Source: CAD feature listing. Evaluate the final solid. Frame: model axes, mm. A direction names the side the tool comes from. Give positions to 0.01 mm unless a question says otherwise; leave off trailing zeros. Loops run counter-clockwise (first coordinate to the right, second up) from the corner with the lowest first, then second, coordinate; pieces in that order, holes last.
from build123d import *

# Parameters (mm, degrees)
SKETCH1_R               = 1.55
BOSS_EXTRUDE1_DEPTH     = 7
SKETCH2_R               = 2.75
CUT_EXTRUDE1_DEPTH      = 5
SKETCH3_R               = 1.75
CUT_EXTRUDE2_DEPTH      = 5
CUT_EXTRUDE4_DEPTH      = 7
CUT_EXTRUDE4_DEPTH_BACK = 7
FILLET1_R               = 10


with BuildPart() as part:
    # Sketch1 → Boss-Extrude1 (new body)
    with BuildSketch(Plane.XY):
        with BuildLine():
            ThreePointArc((0, 6), (-6, 0), (0, -6))
            Line((0, -6), (44.5, -4))
            ThreePointArc((44.5, -4), (48.5, 0), (44.5, 4))
            Line((44.5, 4), (0, 6))
        make_face()
        with Locations((44.5, 0)):
            Circle(SKETCH1_R, mode=Mode.SUBTRACT)
    extrude(amount=BOSS_EXTRUDE1_DEPTH)

    # Sketch2 → Cut-Extrude1 (cut)
    with BuildSketch(Plane.XY.offset(7)):
        Circle(SKETCH2_R)
    extrude(amount=-CUT_EXTRUDE1_DEPTH, mode=Mode.SUBTRACT)

    # Sketch3 → Cut-Extrude2 (cut)
    with BuildSketch(Plane(origin=(0, 0, 0), x_dir=(-1, 0, 0), z_dir=(0, 0, -1))):
        Circle(SKETCH3_R)
    extrude(amount=-CUT_EXTRUDE2_DEPTH, mode=Mode.SUBTRACT)

    # Sketch5 → Cut-Extrude4 (cut, two sides)
    with BuildSketch(Plane(origin=(0, 0, 0), x_dir=(1, 0, 0), z_dir=(0, 1, 0))) as cut_extrude4_sk:
        with BuildLine():
            Line((48.5, 0), (48.5, -2.5))
            Line((48.5, -2.5), (28.5, -2.5))
            add(Edge.make_bspline(
                [(9, 0), (9.734542775, -1.732075598), (8.772191405, -2.578671179), (28.5, -2.5)],
                knots=[0, 0, 0, 0, 1, 1, 1, 1], degree=3))
            Line((9, 0), (48.5, 0))
        make_face()
    extrude(amount=CUT_EXTRUDE4_DEPTH, mode=Mode.SUBTRACT)
    extrude(cut_extrude4_sk.sketch, amount=-CUT_EXTRUDE4_DEPTH_BACK, mode=Mode.SUBTRACT)

    # Fillet1
    fillet1_edges = [part.edges().sort_by_distance(p)[0] for p in [
        (9, 2.797752809, 0),
    ]]
    fillet(fillet1_edges, radius=FILLET1_R)


solid = part.part
1) Cut plane C-C (x = 33). Return loops of the section in (y, z), and give its area (3 significant figures).
Checks:
outline: (-4.52, 2.5) - (4.52, 2.5) - (4.52, 7) - (-4.52, 7) - close
area: 40.7 mm2
2) Cut plane A-A (z = 4.25). Return loops of the section in (x, y).
Checks:
outline: (0, -6) - (44.5, -4) arc R4 ccw to (44.5, 4) - (0, 6) arc R6 ccw to start; hole circle Ø5.5 at (0, 0); hole circle Ø3.1 at (44.5, 0)
3) Contact query for flat-ended pins moving along their axis: P1, Ø4.5, axis at x = 36, y = -0.5, coming from the -Z side; P2, Ø6, axis at x = 1.5, y = 1, coming from the +Z side; P3, Ø1.5, axis at x = 20, y = 0.5, coming from the -Z side; P4, Ø2, axis at x = 32, z = 2.5, coming from the +Y side. Output: stop coordinate, or through.
Checks:
P1: stops at z = 2.5
P2: stops at z = 7
P3: stops at z = 2.44
P4: stops at y = 4.61
4) Pull-direction query (X, two-part tool) for faces 1 (the flat face through (21, 0, 7)), 2 (the cylindrical face through (-6, 0, 3)), 3 (the cylindrical face through (-0.596, -2.685, 4.535)); classes: released by +X, released by -X, zero draft, split by the parting line, or undercut.
Checks:
face 1: zero draft
face 2: released by -X
face 3: undercut
5) Cut plane B-B (x = 42). Return loops of the section in (y, z), and give its area (3 significant figures).
Checks:
outline: (-4.11, 2.5) - (4.11, 2.5) - (4.11, 7) - (-4.11, 7) - close
area: 37.0 mm2
6) Ray query, probe 1 along Y at (x, z) = (44.5, 5.15); probe 2 along X at (y, z) = (-0.25, 6.5); probe 3 along X at (y, z) = (-1.25, 4.25). Return the intervals inside material, ascending.
Checks:
probe 1: y = -4 to -1.55, 1.55 to 4
probe 2: x = -5.99 to -2.74, 2.74 to 42.97, 46.03 to 48.49
probe 3: x = -5.87 to -2.45, 2.45 to 43.58, 45.42 to 48.3
7) Reachability of faces 4 (the cylindrical face through (45.978, 0.466, 4.719)), 5 (the flat face through (36, 0, 2.5)), 6 (the flat face through (2, 0, 2)) from +Z, -Z, +X, -X, +Y, -Y: full face, straight path, thin tool, end or side. Return the list, or none.
Checks:
face 4: +Z, -Z
face 5: -Z, +X, +Y, -Y
face 6: +Z
